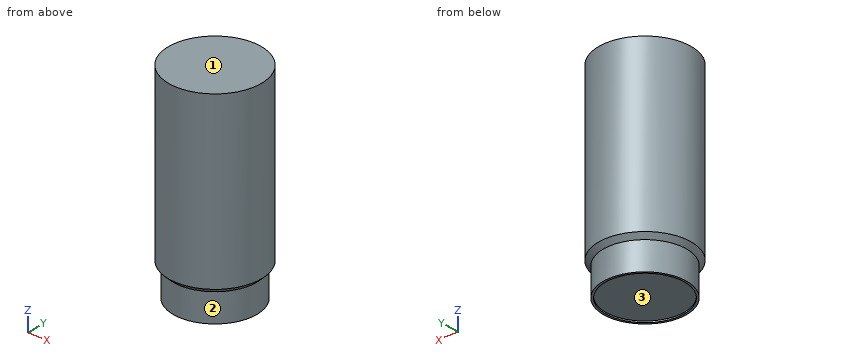
from build123d import *

# Parameters (mm, degrees)
SKETCH2_R          = 5.6
CUT_EXTRUDE1_DEPTH = 0.2


with BuildPart() as part:
    # Sketch1 → Revolve1 (revolve)
    with BuildSketch(Plane(origin=(0, 0, 0), x_dir=(0, 0, -1), z_dir=(1, 0, 0))):
        Polygon((0, 0), (0, 6.55), (24.25, 6.55), (24.9, 5.9), (28.9, 5.9), (28.9, 0), align=None)
    revolve(axis=Axis((0, 0, 0), (0, 0, -1)))

    # Sketch2 → Cut-Extrude1 (cut)
    with BuildSketch(Plane(origin=(0, 0, -28.9), x_dir=(-1, 0, 0), z_dir=(0, 0, -1))):
        Circle(SKETCH2_R)
    extrude(amount=-CUT_EXTRUDE1_DEPTH, mode=Mode.SUBTRACT)


solid = part.part
Geometry: final body of the model. Coordinates: model frame, mm. Face numbers are marked on the shaded views. Give positions to 0.01 mm unless a question says otherwise; leave off trailing zeros. Loops run counter-clockwise (first coordinate to the right, second up) from the corner with the lowest first, then second, coordinate; pieces in that order, holes last. Notation, with made-up numbers: (-24, -39.5) -> (27, -39.5) arc R17 cw to (27, -13.5) -> close; hole circle Ø3 at (62.5, -3.75). An arc over 180 degrees is marked (long way). Put each result on its own line as item: value.
1. Pull-direction query (X, two-part tool) for the marked faces 1, 2 and 3; classes: released by +X, released by -X, zero draft, split by the parting line, or undercut.
Taken from the geometry:
face 1: zero draft
face 2: split by the parting line
face 3: undercut
2. Cut plane C-C (z = -20.75). Return the cut outline in (x, y).
Taken from the geometry:
outline: circle Ø13.1 at (0, 0)
3. Ray query, line 1 along Z through (x, y) = (5.25, 1); line 2 along X through (y, z) = (0.25, -5.25); line 3 along X through (y, z) = (-2.25, -12.25). Return the intervals inside material, ascending. Write a range as [from, to].
Taken from the geometry:
line 1: z = [-28.7, 0]
line 2: x = [-6.55, 6.55]
line 3: x = [-6.15, 6.15]
4. Pin query (flat end, axial travel): P1, Ø2, axis at x = 2.5, y = 3, coming from the -Z side; P2, Ø2, axis at x = -5, z = -19, coming from the +Y side. Return the tip coordinate at first contact, or that it passes through.
Taken from the geometry:
P1: stops at z = -28.7
P2: stops at y = 5.19
5. Cut plane A-A (y = 0). Return the cut outline in (x, z), plus the area to 3 significant figures.
Taken from the geometry:
outline: (-6.55, -24.25) -> (-5.9, -24.9) -> (-5.9, -28.9) -> (-5.6, -28.9) -> (-5.6, -28.7) -> (5.6, -28.7) -> (5.6, -28.9) -> (5.9, -28.9) -> (5.9, -24.9) -> (6.55, -24.25) -> (6.55, 0) -> (-6.55, 0) -> close
area: 371 mm2
